Check sheet for the modelled part. Datum: model origin and axes. Units: mm. A direction names the side the tool comes from. Round coordinates to 2 decimals unless told otherwise and drop trailing zeros. Order: outer loops, then holes, each group sorted by start corner. A loop starts at its lowest first (then second) coordinate and runs counter-clockwise, first axis right, second up. Notation, with made-up numbers: (16.25, 5) -> (30.25, 5) arc R19 ccw to (30.25, 14) -> close; hole circle Ø9 at (-3.75, 36). An arc over 180 degrees is marked (long way). Use CSV: the item, a comma, the result in double quotes.
```python
from build123d import *

# Parameters (mm, degrees)
CROQUIS1_W                          = 11.5
CROQUIS1_H                          = 2.2
CROQUIS2_R                          = 11.4
SALIENTE_EXTRUIR1_DEPTH             = 48
SALIENTE_EXTRUIR2_DEPTH             = 0.4
CORTAR_EXTRUIR1_DEPTH               = 55.027539947
SALIENTE_EXTRUIR3_DEPTH             = 0.4
CORTAR_EXTRUIR2_DEPTH               = 55.027539947
SALIENTE_EXTRUIR4_DEPTH             = 3
CROQUIS8_R                          = 11
SALIENTE_EXTRUIR5_DEPTH             = 25.4
CROQUIS9_R                          = 5
SALIENTE_EXTRUIR6_DEPTH             = 1
CROQUIS10_R                         = 3.5
SALIENTE_EXTRUIR7_DEPTH             = 1.7
SALIENTE_EXTRUIR8_DEPTH             = 9
CROQUIS12_W                         = 1.25
CROQUIS12_H                         = 14
CROQUIS13_W                         = 0.9
CROQUIS13_H                         = 4.4
CROQUIS14_W                         = 0.9
CROQUIS14_H                         = 4.4
CROQUIS15_W                         = 0.9
CROQUIS15_H                         = 4.4
CROQUIS16_W                         = 0.9
CROQUIS16_H                         = 4.4
CROQUIS17_W                         = 0.9
CROQUIS17_H                         = 4.4
CROQUIS18_W                         = 0.9
CROQUIS18_H                         = 4.4
DI_METRO_DE_TALADRO_2_0_2_1_D       = 2
DI_METRO_DE_TALADRO_2_0_2_1_DEPTH   = 7.3
DI_METRO_DE_TALADRO_1_7_1_7_1_D     = 1.7
DI_METRO_DE_TALADRO_1_7_1_7_1_DEPTH = 7.3
DI_METRO_DE_TALADRO_2_2_2_2_1_D     = 2.2
DI_METRO_DE_TALADRO_2_2_2_2_1_DEPTH = 7.3
NERVIO1_START                       = -0.75
NERVIO1_OUTLINE_W                   = 3
NERVIO1_OUTLINE_H                   = 3.2
NERVIO1_DEPTH                       = 1.5
CHAFL_N1_SIZE                       = 0.3


# Read off the part's stored shape, not the designer's step: Nervio1
with BuildPart() as part:
    # Croquis1 → Revolución1 (revolve)
    with BuildSketch(Plane(origin=(0, 0, 0), x_dir=(1, 0, 0), z_dir=(0, 1, 0))):
        with Locations((5.75, -1.1)):
            Rectangle(CROQUIS1_W, CROQUIS1_H)
    revolve(axis=Axis((0, 0, 0), (0, 0, 1)))

    # Croquis2 → Saliente-Extruir1 (add)
    with BuildSketch(Plane(origin=(0, 0, 0), x_dir=(-1, 0, 0), z_dir=(0, 0, -1))):
        with Locations(Location((0, 0, 0), (0, 0, 90))):
            Circle(CROQUIS2_R)
    extrude(amount=SALIENTE_EXTRUIR1_DEPTH)

    # Croquis3 → Saliente-Extruir2 (add)
    with BuildSketch(Plane(origin=(-1.187185199, 0.491748211, 0), x_dir=(0.38268343236508984, 0.9238795325112867, 0), z_dir=(0.9238795325112867, -0.38268343236508984, 0))):
        Polygon((7.1, -51), (8.9, -51), (9.2, -50.7), (9.2, -48), (6.8, -48), (6.8, -50.7), align=None)
    extrude(amount=-SALIENTE_EXTRUIR2_DEPTH)

    # Croquis4 → Cortar-Extruir1 (cut, through all)
    with BuildSketch(Plane(origin=(-1.556737012, 0.644821584, 0), x_dir=(0, 0, 1), z_dir=(-0.9238795325112865, 0.3826834323650905, 0))):
        with BuildLine():
            Line((-51, 8.5), (-51, 7.5))
            Line((-51, 7.5), (-49.8, 7.5))
            ThreePointArc((-49.8, 7.5), (-49.3, 8), (-49.8, 8.5))
            Line((-49.8, 8.5), (-51, 8.5))
        make_face()
    extrude(amount=-CORTAR_EXTRUIR1_DEPTH, mode=Mode.SUBTRACT)

    # Croquis5 → Saliente-Extruir3 (add)
    with BuildSketch(Plane(origin=(1.187185199, -0.491748211, 0), x_dir=(-0.3826834323650898, -0.9238795325112867, 0), z_dir=(-0.9238795325112867, 0.3826834323650898, 0))):
        Polygon((7.1, -51), (8.9, -51), (9.2, -50.7), (9.2, -48), (6.8, -48), (6.8, -50.7), align=None)
    extrude(amount=-SALIENTE_EXTRUIR3_DEPTH)

    # Croquis6 → Cortar-Extruir2 (cut, through all)
    with BuildSketch(Plane(origin=(1.556737012, -0.644821584, 0), x_dir=(0, 0, -1), z_dir=(0.9238795325112837, -0.38268343236509744, -9.353628982466952e-15))):
        with BuildLine():
            Line((51, -7.5), (49.8, -7.5))
            ThreePointArc((49.8, -7.5), (49.3, -8), (49.8, -8.5))
            Line((49.8, -8.5), (51, -8.5))
            Line((51, -8.5), (51, -7.5))
        make_face()
    extrude(amount=-CORTAR_EXTRUIR2_DEPTH, mode=Mode.SUBTRACT)

    # Croquis7 → Saliente-Extruir4 (add)
    with BuildSketch(Plane(origin=(0, 0, -48), x_dir=(-1, 0, 0), z_dir=(0, 0, -1))):
        with BuildLine():
            Line((-4.326858651, 2.699684096), (1.150586162, 4.968516024))
            ThreePointArc((1.150586162, 4.968516024), (4.711785616, 1.951685505), (4.326858651, -2.699684096))
            Line((4.326858651, -2.699684096), (-1.150586162, -4.968516024))
            ThreePointArc((-1.150586162, -4.968516024), (-4.711785616, -1.951685505), (-4.326858651, 2.699684096))
        make_face()
    extrude(amount=SALIENTE_EXTRUIR4_DEPTH)

    # Croquis8 → Saliente-Extruir5 (add)
    with BuildSketch(Plane.XY.offset(2.2)):
        Circle(CROQUIS8_R)
    extrude(amount=SALIENTE_EXTRUIR5_DEPTH)

    # Croquis9 → Saliente-Extruir6 (add)
    with BuildSketch(Plane.XY.offset(27.6)):
        Circle(CROQUIS9_R)
    extrude(amount=SALIENTE_EXTRUIR6_DEPTH)

    # Croquis10 → Saliente-Extruir7 (add)
    with BuildSketch(Plane.XY.offset(28.6)):
        Circle(CROQUIS10_R)
    extrude(amount=SALIENTE_EXTRUIR7_DEPTH)

    # Croquis11 → Saliente-Extruir8 (add)
    with BuildSketch(Plane.XY.offset(30.3)):
        with BuildLine():
            Line((-0.660243548, 1.897070133), (1.784111936, 0.88458494))
            ThreePointArc((1.784111936, 0.88458494), (-0.777457819, -1.842750828), (-0.660243548, 1.897070133))
        make_face()
    extrude(amount=SALIENTE_EXTRUIR8_DEPTH)

    # Croquis12 → Revolución2 (revolve)
    with BuildSketch(Plane(origin=(0, 0, 0), x_dir=(1, 0, 0), z_dir=(0, 1, 0))):
        with Locations((0.625, 58)):
            Rectangle(CROQUIS12_W, CROQUIS12_H)
    revolve(axis=Axis((0, 0, -65), (0, 0, 1)))

    # Croquis13 → Cortar-Revolución1 (revolve, cut)
    with BuildSketch(Plane(origin=(0, -7.852976026, 0), x_dir=(1, 0, 0), z_dir=(0, 1, 0))):
        with Locations((3.702809175, 2.2)):
            Rectangle(CROQUIS13_W, CROQUIS13_H)
    revolve(axis=Axis((3.252809175, -7.852976026, -4.4), (0, 0, 1)), mode=Mode.SUBTRACT)

    # Croquis14 → Cortar-Revolución2 (revolve, cut)
    with BuildSketch(Plane(origin=(0, 2.678784027, 0), x_dir=(1, 0, 0), z_dir=(0, 1, 0))):
        with Locations((6.917156728, 2.2)):
            Rectangle(CROQUIS14_W, CROQUIS14_H)
    revolve(axis=Axis((6.467156728, 2.678784027, -4.4), (0, 0, 1)), mode=Mode.SUBTRACT)

    # Croquis15 → Cortar-Revolución3 (revolve, cut)
    with BuildSketch(Plane(origin=(0, -2.678784027, 0), x_dir=(1, 0, 0), z_dir=(0, 1, 0))):
        with Locations((-6.017156728, 2.2)):
            Rectangle(CROQUIS15_W, CROQUIS15_H)
    revolve(axis=Axis((-6.467156728, -2.678784027, -4.4), (0, 0, 1)), mode=Mode.SUBTRACT)

    # Croquis16 → Cortar-Revolución4 (revolve, cut)
    with BuildSketch(Plane(origin=(0, 6.743503392, 0), x_dir=(1, 0, 0), z_dir=(0, 1, 0))):
        with Locations((5.624472147, 2.2)):
            Rectangle(CROQUIS16_W, CROQUIS16_H)
    revolve(axis=Axis((5.174472147, 6.743503392, -4.4), (0, 0, 1)), mode=Mode.SUBTRACT)

    # Croquis17 → Cortar-Revolución5 (revolve, cut)
    with BuildSketch(Plane(origin=(0, 1.109472634, 0), x_dir=(1, 0, 0), z_dir=(0, 1, 0))):
        with Locations((-7.977281322, 2.2)):
            Rectangle(CROQUIS17_W, CROQUIS17_H)
    revolve(axis=Axis((-8.427281322, 1.109472634, -4.4), (0, 0, 1)), mode=Mode.SUBTRACT)

    # Croquis18 → Cortar-Revolución6 (revolve, cut)
    with BuildSketch(Plane(origin=(0, 7.852976026, 0), x_dir=(1, 0, 0), z_dir=(0, 1, 0))):
        with Locations((-2.802809175, 2.2)):
            Rectangle(CROQUIS18_W, CROQUIS18_H)
    revolve(axis=Axis((-3.252809175, 7.852976026, -4.4), (0, 0, 1)), mode=Mode.SUBTRACT)

    # Diámetro de taladro Ø2.0 (2)1
    with Locations(Plane.XY.offset(27.6)):
        with Locations((-3.5, -6.062177826), (7, 0)):
            Hole(DI_METRO_DE_TALADRO_2_0_2_1_D / 2, depth=DI_METRO_DE_TALADRO_2_0_2_1_DEPTH)

    # Diámetro de taladro Ø1.7 (1.7)1
    with Locations(Plane.XY.offset(27.6)):
        with Locations((9.5, 0), (-4.75, 8.227241336), (-4.75, -8.227241336)):
            Hole(DI_METRO_DE_TALADRO_1_7_1_7_1_D / 2, depth=DI_METRO_DE_TALADRO_1_7_1_7_1_DEPTH)

    # Diámetro de taladro Ø2.2 (2.2)1
    with Locations(Plane.XY.offset(27.6)):
        with Locations((4.25, 7.361215932), (-8.5, 0), (-3.5, 6.062177826), (4.25, -7.361215932)):
            Hole(DI_METRO_DE_TALADRO_2_2_2_2_1_D / 2, depth=DI_METRO_DE_TALADRO_2_2_2_2_1_DEPTH)

    # Nervio1 outline → Nervio1 (add)
    with BuildSketch(Plane(origin=(0, 0, 0), x_dir=(0.38268343236508995, -0.9238795325112867, 0), z_dir=(-0.9238795325112867, -0.38268343236508995, 0)).offset(NERVIO1_START)):
        with Locations((-5.5, -48.6)):
            Rectangle(NERVIO1_OUTLINE_W, NERVIO1_OUTLINE_H)
    extrude(amount=NERVIO1_DEPTH)

    # Chaflán1
    chafl_n1_edges = [part.edges().sort_by_distance(p)[0] for p in [
        (-1.25, 0, -65),
    ]]
    chamfer(chafl_n1_edges, length=CHAFL_N1_SIZE)


solid = part.part
```
Q1. Sectioned sample at A-A, the plane z = 26. State how many separate pieces and enclosed holes the cut face has, then the cut area to 3 significant figures.
Result sheet:
separate pieces,"1"
enclosed holes,"9"
area,"352 mm^2"
Q2. Access from +Z, -Z, +X, -X, +Y, -Y to the whole of each face (thin tool, end or side, straight path). Record for faces 4 (the face through (7.299, 2.334, -2.231)), 5 (the face through (4.685, -2.014, -49.479)), 6 (the face through (-4.5, 5.6, 23.9)).
Result sheet:
face 4,"none"
face 5,"-Z, +X"
face 6,"+Z"
Q3. Mould release check, pull along X, two halves, no side actions. Record for faces 1 (the face through (-7, -9, -24)), 2 (the face through (2.2, -3.3, 28.6)), 3 (the face through (10, 0, 20.3)): pulls with the +X half, pulls with the -X half, needs draft (parallel to the pull), parting line crosses it, or undercut.
Result sheet:
face 1,"parting line crosses it"
face 2,"needs draft"
face 3,"undercut"
Q4. Sectioned sample at C-C, the plane z = 6.5. Enter the section's corners in (x, y), then the cut area to 3 significant figures.
Result sheet:
outline,"circle Ø22 at (0, 0)"
area,"380 mm^2"
Q5. Scan lines: L1, parallel to Y at x = -3.5, z = 23.75; L2, parallel to Z at x = 8.25, y = -3.5; L3, parallel to Y at x = -0.25, z = -29.5. Record each from-to range of solid material in increasing order.
Result sheet:
L1,"y = -10.43 to -7.06, -5.06 to 4.96, 7.16 to 10.43"
L2,"z = -48 to 27.6"
L3,"y = -11.4 to 11.4"
Q6. Go/stop test with flat-tipped pins: pin 1 (2 mm diameter, centred on y = 6, z = 16, fed in from +X); pin 2 (1.1 mm diameter, centred on x = -2, y = 5, fed in from -Z); pin 3 (0.5 mm diameter, centred on x = 6.5, y = 3, fed in from -Z). Record where each tip stops, or that it passes through.
Result sheet:
pin 1,"stops at x = 9.8"
pin 2,"stops at z = -51"
pin 3,"stops at z = -48"
Q7. Sectioned sample at B-B, the plane z = -42. Enter the section's corners in (x, y).
Result sheet:
outline,"circle Ø22.8 at (0, 0)"
